```python
from build123d import *

# Parameters (mm, degrees)
F1_DEPTH = 30
F2_R     = 1.65
F3_DEPTH = 3.001
F4_R     = 2
F5_DEPTH = 3.001


with BuildPart() as f1:
    # F0 (on Top) → F1 (new body)
    with BuildSketch(Plane.XY):
        Polygon((0, 25), (0, 0), (15, 0), (15, 3), (3, 3), (3, 25), align=None)
    extrude(amount=F1_DEPTH)

    # F2 (on face) → F3 (cut, through all)
    with BuildSketch(Plane.YZ.offset(3)):
        with Locations((22, 4)):
            Circle(F2_R)
        with Locations((11.7, 26.2)):
            Circle(F2_R)
    extrude(amount=-F3_DEPTH, mode=Mode.SUBTRACT)

    # F4 (on face) → F5 (cut, through all)
    with BuildSketch(Plane(origin=(0, 3, 0), x_dir=(-1, 0, 0), z_dir=(0, 1, 0))):
        with Locations((-9, 24)):
            Circle(F4_R)
        with Locations((-9, 6)):
            Circle(F4_R)
    extrude(amount=-F5_DEPTH, mode=Mode.SUBTRACT)


solid = f1.part
```
Input: part model. Units: mm. Frame: model coordinates. A direction names the side the tool comes from. Give positions to 0.01 mm unless a question says otherwise; leave off trailing zeros. Loops run counter-clockwise (first coordinate to the right, second up) from the corner with the lowest first, then second, coordinate; pieces in that order, holes last.
1) Section query D-D on x = 2. Return the cut outline in (y, z).
A:
outline: (0, 0) - (25, 0) - (25, 30) - (0, 30) - close; hole circle Ø3.3 at (11.7, 26.2); hole circle Ø3.3 at (22, 4)
2) Line query: L1, parallel to Z at x = 9, y = 2; L2, parallel to Z at x = 1, y = 11.7; L3, parallel to Z at x = 0.9, y = 22. Output: solid intervals per line, ascending.
A:
L1: z = 0 to 4, 8 to 22, 26 to 30
L2: z = 0 to 24.55, 27.85 to 30
L3: z = 0 to 2.35, 5.65 to 30
3) Section query A-A on z = 24. Return the cut outline in (x, y).
A:
outline: (0, 0) - (7, 0) - (7, 3) - (3, 3) - (3, 25) - (0, 25) - close; (11, 0) - (15, 0) - (15, 3) - (11, 3) - close
4) Mould query, pull axis Z, two halves, no side actions, for faces 1 (the flat face through (2, 11, 0)), 2 (the cylindrical face through (9, 2, 8)), 3 (the flat face through (0, 13, 15)). Classes: released by +Z, released by -Z, zero draft, split by the parting line, or undercut.
A:
face 1: released by -Z
face 2: undercut
face 3: zero draft
5) Contact query for flat-ended pins moving along their axis: pin 1 (2 mm diameter, centred on y = 11.7, z = 26.2, fed in from -X); pin 2 (4.5 mm diameter, centred on x = 9, z = 24, fed in from +Y); pin 3 (8 mm diameter, centred on y = 15.5, z = 7.5, fed in from +X). Output: stop coordinate, or through.
A:
pin 1: passes through
pin 2: stops at y = 3
pin 3: stops at x = 3
6) Reachability of faces 4 (the cylindrical face through (1.52, 20.35, 4.07)), 5 (the flat face through (3, 14, 15)) from +Z, -Z, +X, -X, +Y, -Y: full face, straight path, thin tool, end or side. Return the list, or none.
A:
face 4: +X, -X
face 5: +Z, -Z, +X, +Y
7) Section query B-B on x = 9. Return the cut outline in (y, z), and give its area (3 significant figures).
A:
outline: (0, 0) - (3, 0) - (3, 4) - (0, 4) - close; (0, 8) - (3, 8) - (3, 22) - (0, 22) - close; (0, 26) - (3, 26) - (3, 30) - (0, 30) - close
area: 66.0 mm2
8) Section query C-C on y = 13. Return the cut outline in (x, z), and give its area (3 significant figures).
A:
outline: (0, 0) - (3, 0) - (3, 25.18) - (0, 25.18) - close; (0, 27.22) - (3, 27.22) - (3, 30) - (0, 30) - close
area: 83.9 mm2
